Part model, mm, in its own coordinate system. Face numbers are marked on the shaded views. A direction names the side the tool comes from. Round coordinates to 2 decimals unless told otherwise and drop trailing zeros. Order: outer loops, then holes, each group sorted by start corner. A loop starts at its lowest first (then second) coordinate and runs counter-clockwise, first axis right, second up. Notation, with made-up numbers: M 51,-7.5 L 104,-7.5 A15 cw 104,-3.5 Z; hole C 66.25,71.5 d5. An arc over 180 degrees is marked long. Write each question's results on one line, items separated by ' | '. Start each with the question number.
1. Probe L1, parallel to Y at x = 3.5, z = -11; L2, parallel to Y at x = -9.25, z = -7.75; L3, parallel to Z at x = -1, y = 2.25. List the from-to ranges inside material, lowest first. Write a range as [from, to].
2. Band-saw the part on D-D, the plane y = 5. List the corners of the cut face in (x, z).
3. Band-saw the part on C-C, the plane y = 2.75. List the corners of the cut face in (x, z).
4. Drop a flat-ended pin along its axis: pin 1 Ø4 at (x, y) = (11, 1.5) entering from +Z. Give the stop position or say it passes through.
5. Which spindle directions (+Z, -Z, +X, -X, +Y, -Y) get a long thin tool onto all of the face, cutting with end or side? Do the marked faces 1 and 2. Say none if no direction does.
6. Two-plate mould, pull along X, no slides. Class the marked faces 3, 4 and 5: +X half, -X half, draft (parallel to the pull), parting line (faces both ways), or undercut.
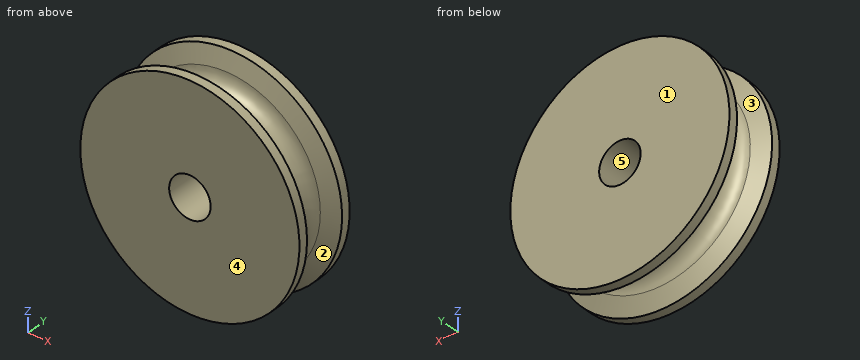
```python
from build123d import *

# Parameters (mm, degrees)
SKETCH1_R           = 14
SKETCH1_R_2         = 2.65
BOSS_EXTRUDE1_DEPTH = 6
CUT_EXTRUDE1_START  = -4
SKETCH2_R           = 14
SKETCH2_R_2         = 10
CUT_EXTRUDE1_DEPTH  = 4
SKETCH3_R           = 14
SKETCH3_R_2         = 2.65
BOSS_EXTRUDE2_DEPTH = 2
FILLET1_R           = 2


with BuildPart() as part:
    # Sketch1 → Boss-Extrude1 (new body)
    with BuildSketch(Plane(origin=(0, 0, 0), x_dir=(1, 0, 0), z_dir=(0, 1, 0))):
        with Locations(Location((0, 0, 0), (0, 0, 270))):
            Circle(SKETCH1_R)
        with Locations(Location((0, 0, 0), (0, 0, 270))):
            Circle(SKETCH1_R_2, mode=Mode.SUBTRACT)
    extrude(amount=BOSS_EXTRUDE1_DEPTH)

    # Sketch2 → Cut-Extrude1 (cut)
    with BuildSketch(Plane(origin=(0, 6, 0), x_dir=(1, 0, 0), z_dir=(0, 1, 0)).offset(CUT_EXTRUDE1_START)):
        with Locations(Location((0, 0, 0), (0, 0, 270))):
            Circle(SKETCH2_R)
        with Locations(Location((0, 0, 0), (0, 0, 270))):
            Circle(SKETCH2_R_2, mode=Mode.SUBTRACT)
    extrude(amount=CUT_EXTRUDE1_DEPTH, mode=Mode.SUBTRACT)

    # Sketch3 → Boss-Extrude2 (add)
    with BuildSketch(Plane(origin=(0, 6, 0), x_dir=(1, 0, 0), z_dir=(0, 1, 0))):
        with Locations(Location((0, 0, 0), (0, 0, 270))):
            Circle(SKETCH3_R)
        with Locations(Location((0, 0, 0), (0, 0, 270))):
            Circle(SKETCH3_R_2, mode=Mode.SUBTRACT)
    extrude(amount=BOSS_EXTRUDE2_DEPTH)

    # Fillet1
    fillet1_edges = [part.edges().sort_by_distance(p)[0] for p in [
        (0, 2, -10),
        (0, 6, -10),
    ]]
    fillet(fillet1_edges, radius=FILLET1_R - 0.0001)  # a hair under: the kernel refuses the full size

    # Chamfer1: read off the stored shape, not the designer's step
    # Chamfer1 outline → Chamfer1 (revolve, cut)
    with BuildSketch(Plane.XY):
        Polygon((11.858584332, 5.994994138), (12, 5.994994138), (12, 6), (14, 6), (14, 6.792991793), align=None)
        Polygon((12, 2.005005862), (11.858584332, 2.005005862), (14, 1.207008207), (14, 2), (12, 2), align=None)
    revolve(axis=Axis((0, 0, 0), (0, 1, 0)), mode=Mode.SUBTRACT)


solid = part.part
```
Solution:
1) L1: [0, 2.05], [5.95, 8] | L2: [0, 1.93], [6.07, 8] | L3: [-10.99, -2.45], [2.45, 10.99]
2) outline: C 0,0 d20.54; hole C 0,0 d5.3
3) outline: C 0,0 d20.88; hole C 0,0 d5.3
4) pin 1: z = 10.71
5) face 1: +Z, -Z, +X, -X, +Y | face 2: none
6) face 3: parting line | face 4: draft | face 5: undercut
